Study the drawing (mm; zero at the part's minimum x, y, z) and answer. Round coordinates to 2 decimals unless told otherwise and drop trailing zeros. Write each loop counter-clockwise with the first axis right and the second up, starting at its lowest first coordinate (ties: lowest second). Pieces come first, ordered by that corner, then holes. Notation, with made-up numbers: (14, 30) - (62, 30) arc R5 cw to (62, 38) - close; hole circle Ø5 at (-20.5, 22.25). An arc over 180 degrees is marked (long way). Return JSON: item names as keys, results as strings. Group by question number.
(1) This flat-tipped pin is pushed along its axis until it touches: pin 1 (0.6 mm diameter, centred on y = 29.5, z = 21.5, fed in from -X). Where does it stop, or does it pass through?
(2) Section C-C, the plane z = 22.5 is taken. Write down the section's boundary in (x, y).
(3) Section B-B, the plane y = 11.5 is taken. Write down the section's boundary in (x, z), then the cut area to 3 significant figures.
(4) Section D-D, the plane z = 5 is taken. Write down the section's boundary in (x, y).
(5) Find the intervals of material crossed by line 1 along Z through (x, y) = (2.35, 15); line 2 along Z through (x, y) = (3.9, 22.5); line 3 along Y through (x, z) = (1.1, 4.5), in increasing order. Write a range as [from, to].
(6) Section A-A, the plane x = 0.5 is taken. Write down the section's boundary in (y, z).
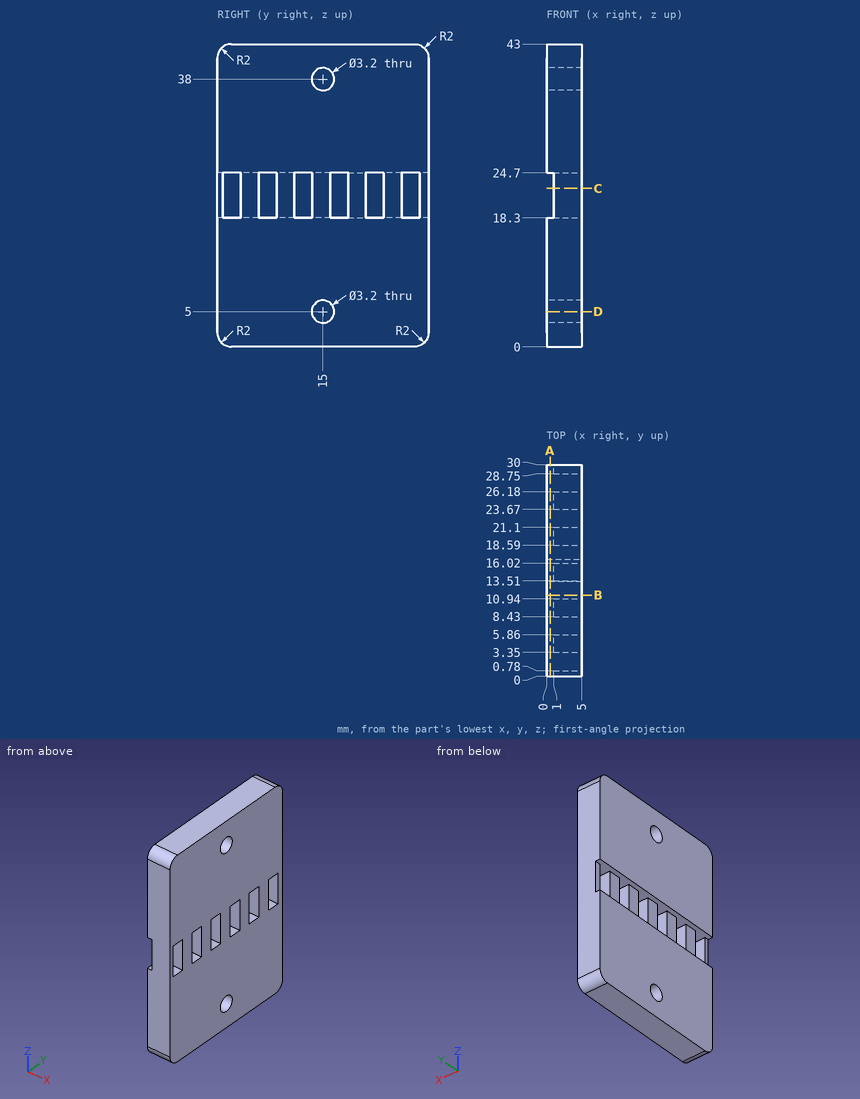
Working result:
{
 "1": {"pin 1": "stops at x = 1"},
 "2": {"outline": "(1, 0) - (5, 0) - (5, 0.78) - (1, 0.78) - close; (1, 3.35) - (5, 3.35) - (5, 5.86) - (1, 5.86) - close; (1, 8.43) - (5, 8.43) - (5, 10.94) - (1, 10.94) - close; (1, 13.51) - (5, 13.51) - (5, 16.02) - (1, 16.02) - close; (1, 18.59) - (5, 18.59) - (5, 21.1) - (1, 21.1) - close; (1, 23.67) - (5, 23.67) - (5, 26.18) - (1, 26.18) - close; (1, 28.75) - (5, 28.75) - (5, 30) - (1, 30) - close"},
 "3": {"outline": "(0, 0) - (5, 0) - (5, 18.3) - (0, 18.3) - close; (0, 24.7) - (5, 24.7) - (5, 43) - (0, 43) - close", "area": "183 mm^2"},
 "4": {"outline": "(0, 0) - (5, 0) - (5, 13.4) - (0, 13.4) - close; (0, 16.6) - (5, 16.6) - (5, 30) - (0, 30) - close"},
 "5": {"line 1": "z = [0, 3.4], [6.6, 36.4], [39.6, 43]", "line 2": "z = [0, 18.3], [24.7, 43]", "line 3": "y = [0, 13.48], [16.52, 30]"},
 "6": {"outline": "(0, 2) arc R2 ccw to (2, 0) - (28, 0) arc R2 ccw to (30, 2) - (30, 18.3) - (0, 18.3) - close; (0, 24.7) - (30, 24.7) - (30, 41) arc R2 ccw to (28, 43) - (2, 43) arc R2 ccw to (0, 41) - close; hole circle Ø3.2 at (15, 5); hole circle Ø3.2 at (15, 38)"}
}
